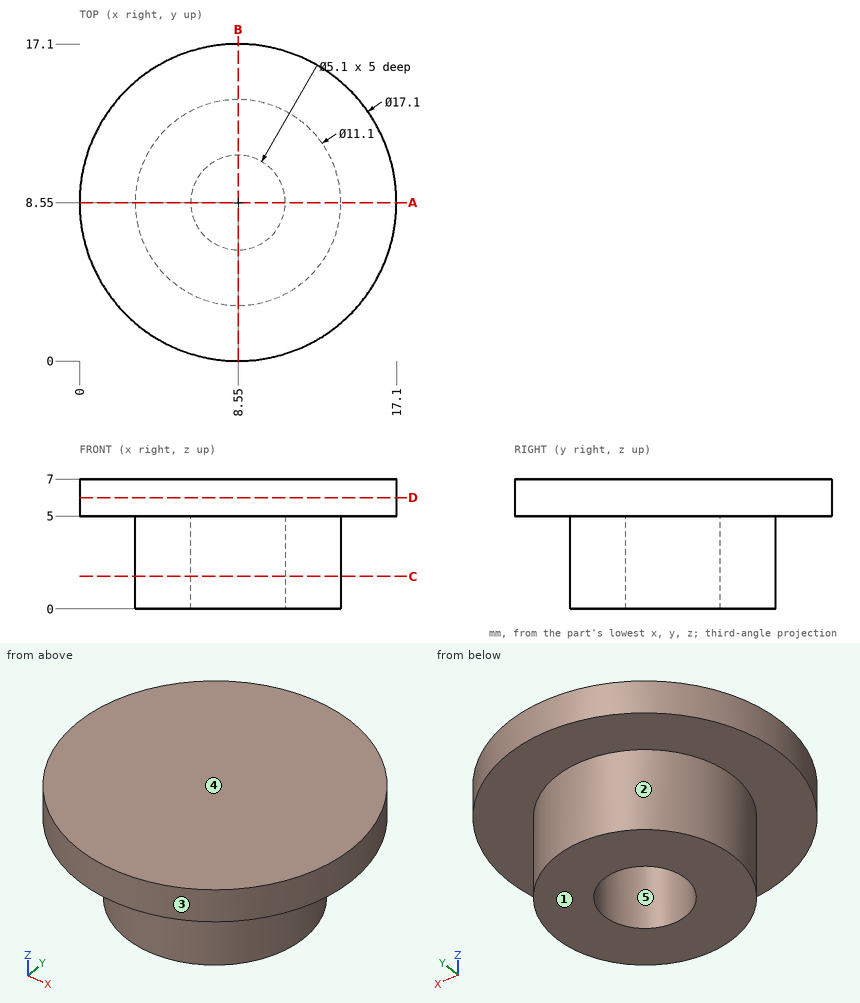
Here's the drawing with two shaded views (mm, measured from the low corner). I have some questions. A direction names the side the tool comes from. Coordinates: 2 decimals unless noted, no trailing zeros. Order: outer loops, then holes, each group sorted by start corner. A loop starts at its lowest first (then second) coordinate and runs counter-clockwise, first axis right, second up.
Q1. Will these pins go through, and if not, where does the flat tip stop? pin 1 (3 mm diameter, centred on x = 3.5, z = 6, fed in from -Y); pin 2 (1.5 mm diameter, centred on y = 7.5, z = 2, fed in from +X); pin 3 (1 mm diameter, centred on x = 5, z = 1.5, fed in from -Y).
Q2. Which directions (+Z, -Z, +X, -X, +Y, -Y) give clear straight access to the entire face, cutting with the end or side of a thin tool? Please do the marked faces 1 and 2.
Q3. Thinking about a two-plate mould opening in Y: for the marked faces 3, 4 and 5, which applies, released by +Y, released by -Y, zero draft, split by the parting line, or undercut?
Q4. Suppose I cut it at A-A on y = 8.55. Please give me the cut outline in (x, z).
Q5. Suppose I cut it at D-D on z = 6. Please give me the cut outline in (x, y), and give its area (3 significant figures).
Q6. Please list where these lines run through material, in increasing order: L1, parallel to Y at x = 8.55, z = 3.95; L2, parallel to Z at x = 15.25, y = 13; L3, parallel to Y at x = 7, z = 2.75.
Q7. Suppose I cut it at C-C on z = 1.75. Please give me the cut outline in (x, y), and give its area (3 significant figures).
Answer:
1. pin 1: stops at y = 0.77
1. pin 2: stops at x = 14.09
1. pin 3: stops at y = 3.91
2. face 1: -Z, +X, -X, +Y, -Y
2. face 2: -Z
3. face 3: split by the parting line
3. face 4: zero draft
3. face 5: undercut
4. outline: (0, 5) - (3, 5) - (3, 0) - (6, 0) - (6, 5) - (11.1, 5) - (11.1, 0) - (14.1, 0) - (14.1, 5) - (17.1, 5) - (17.1, 7) - (0, 7) - close
5. outline: circle Ø17.1 at (8.55, 8.55)
5. area: 230 mm2
6. L1: y = 3 to 6, 11.1 to 14.1
6. L2: z = 5 to 7
6. L3: y = 3.22 to 6.53, 10.57 to 13.88
7. outline: circle Ø11.1 at (8.55, 8.55); hole circle Ø5.1 at (8.55, 8.55)
7. area: 76.3 mm2
